Answer from the drawing. Dimensions are ordinates in mm from the lowest x, y and z of the part. A direction names the side the tool comes from. Give positions to 0.01 mm unless a question says otherwise; leave off trailing zeros. Loops run counter-clockwise (first coordinate to the right, second up) from the corner with the lowest first, then second, coordinate; pieces in that order, holes last. Notation, with made-up numbers: (34, 37) - (74, 37) arc R15 cw to (74, 58) - close; hole circle Ø1 at (37, 77.25). An arc over 180 degrees is marked (long way). One line per item, written item: value.
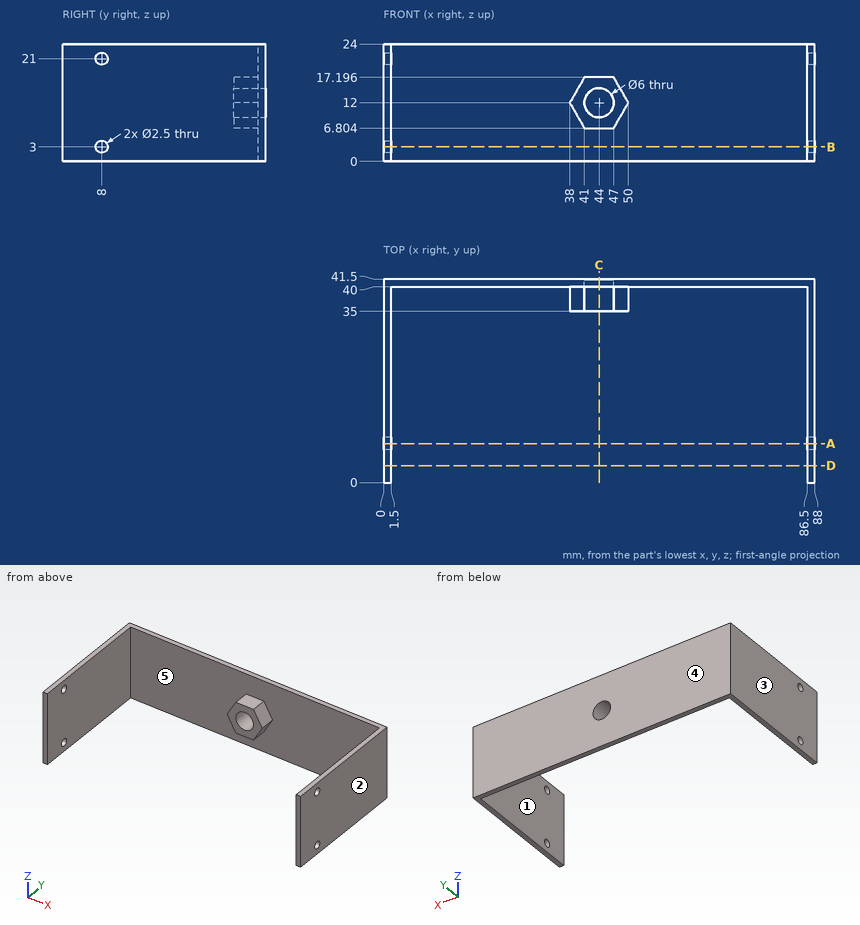
1. Section C-C (x = 44) is taken. Write down the section's boundary in (y, z).
Output:
outline: (35, 6.8) - (40, 6.8) - (40, 0) - (41.5, 0) - (41.5, 9) - (35, 9) - close; (35, 15) - (41.5, 15) - (41.5, 24) - (40, 24) - (40, 17.2) - (35, 17.2) - close
2. For the marked faces 1 and 2, determine the directions among +Z, -Z, +X, -X, +Y, -Y from which every point of the face is accessible in a straight line to the end or side of a thin tool.
Output:
face 1: +Z, -Z, -Y
face 2: +Z, -Z, +X, +Y, -Y
3. Section A-A (y = 8) is taken. Write down the section's boundary in (x, z).
Output:
outline: (0, 0) - (1.5, 0) - (1.5, 1.75) - (0, 1.75) - close; (0, 4.25) - (1.5, 4.25) - (1.5, 19.75) - (0, 19.75) - close; (0, 22.25) - (1.5, 22.25) - (1.5, 24) - (0, 24) - close; (86.5, 0) - (88, 0) - (88, 1.75) - (86.5, 1.75) - close; (86.5, 4.25) - (88, 4.25) - (88, 19.75) - (86.5, 19.75) - close; (86.5, 22.25) - (88, 22.25) - (88, 24) - (86.5, 24) - close
4. Section B-B (z = 3) is taken. Write down the section's boundary in (x, y).
Output:
outline: (0, 0) - (1.5, 0) - (1.5, 6.75) - (0, 6.75) - close; (0, 9.25) - (1.5, 9.25) - (1.5, 40) - (86.5, 40) - (86.5, 9.25) - (88, 9.25) - (88, 41.5) - (0, 41.5) - close; (86.5, 0) - (88, 0) - (88, 6.75) - (86.5, 6.75) - close
5. Section D-D (y = 3.5) is taken. Write down the section's boundary in (x, z).
Output:
outline: (0, 0) - (1.5, 0) - (1.5, 24) - (0, 24) - close; (86.5, 0) - (88, 0) - (88, 24) - (86.5, 24) - close
6. Flat-ended cylindrical pins translate along their axes: pin 1 Ø8.5 at (x, z) = (41.5, 13.5) entering from -Y; pin 2 Ø1.5 at (x, y) = (45, 37) entering from +Z; pin 3 Ø4 at (x, y) = (44, 36.5) entering from -Z. Find the tip coordinate at first contact, or state that the pin passes through.
Output:
pin 1: stops at y = 35
pin 2: stops at z = 17.2
pin 3: stops at z = 6.8
7. The mould has two halves that part along X. Classify the marked faces 3, 4 and 5: released by +X, released by -X, zero draft, split by the parting line, or undercut.
Output:
face 3: released by -X
face 4: zero draft
face 5: undercut
8. Find the intervals of material crossed by line 1 along X through (y, z) = (9, 9.25); line 2 along Y through (x, z) = (0.75, 21); line 3 along Y through (x, z) = (28, 5.5), in increasing order.
Output:
line 1: x = 0 to 1.5, 86.5 to 88
line 2: y = 0 to 6.75, 9.25 to 41.5
line 3: y = 40 to 41.5
